Autodesk Inventor part; units mm, degrees
ref_plane "YZ Plane" through (0, 0, 0) normal (1, 0, 0) x (0, 1, 0)
ref_plane "XZ Plane" through (0, 0, 0) normal (0, 1, 0) x (-1, 0, 0)
ref_plane "XY Plane" through (0, 0, 0) normal (0, 0, 1) x (1, 0, 0)
sketch "Sketch1" plane through (0, 0, 0) normal (0, 0, 1) x (1, 0, 0)
  line L0 (13.4603, 15.4458) -> (13.4545, -36.9417)
  circle A0 centre (18.2181, -26.6234) radius 2.3812
  circle A1 centre (18.2217, 5.1266) radius 2.3812
  circle A2 centre (78.5467, 5.1199) radius 2.3812
  circle A3 centre (78.5431, -26.6301) radius 2.3812
  circle A4 centre (169.0306, -26.6401) radius 2.3812
  circle A5 centre (229.3556, -26.6468) radius 2.3812
  circle A6 centre (229.3592, 5.1032) radius 2.3812
  line L1 (234.1228, 15.4214) -> (234.117, -36.9661)
  circle A7 centre (169.0342, 5.1099) radius 2.3812
  line L2 (13.4545, -36.9417) -> (234.117, -36.9661)
  line L3 (234.1228, 15.4214) -> (13.4603, 15.4458)
  point P0 (3.3527, -2.3752)
extrude "Extrusion1" add sketch "Sketch1" along normal blind 12.7
sketch "Sketch3" plane through (0, 0, 0) normal (0, 0, -1) x (-1, 0, 0)
  line L0 (-234.117, -36.9661) -> (-234.1228, 15.4214)
  line L1 (-234.1199, -10.7723) -> (-13.4574, -10.7479)
  line L2 (-13.4603, 15.4458) -> (-13.4545, -36.9417)
  line L3 (-234.1228, 15.4214) -> (-13.4603, 15.4458)
  line L4 (-123.7915, 15.4336) -> (-123.7857, -36.9539)
  line L5 (-13.4545, -36.9417) -> (-234.117, -36.9661)
  circle A0 centre (-155.5369, -26.2636) radius 1.5
  circle A1 centre (-131.5369, -26.261) radius 1.5
  circle A2 centre (-155.5404, 4.7364) radius 1.5
  circle A3 centre (-131.5404, 4.739) radius 1.5
  point P0 (0, 0)
  dimension "d8" = 15.5
  dimension "d9" = 31.75
  dimension "d10" = 3
  dimension "d13" = 24
  dimension "d16" = 31
extrude "Extrusion2" cut sketch "Sketch3" against normal blind 12.7 contours A0 | A1 | A2 | A3
sketch "Sketch4" plane through (0, 0, 0) normal (0, 0, -1) x (-1, 0, 0)
  circle A0 centre (-131.5369, -26.261) radius 1.5
  circle A1 centre (-131.5369, -26.261) radius 3.175
  circle A2 centre (-155.5369, -26.2636) radius 1.5
  circle A3 centre (-155.5369, -26.2636) radius 3.175
  circle A4 centre (-131.5404, 4.739) radius 1.5
  circle A5 centre (-131.5404, 4.739) radius 3.175
  circle A6 centre (-155.5404, 4.7364) radius 1.5
  circle A7 centre (-155.5404, 4.7364) radius 3.175
  point P0 (0, 0)
  dimension "d21" = 6.35
  dimension "d22" = 6.35
  dimension "d23" = 6.35
  dimension "d24" = 6.35
extrude "Extrusion3" cut sketch "Sketch4" against normal blind 3.175
sketch "Sketch5" plane through (0, 0, 0) normal (0, 0, -1) x (-1, 0, 0)
  point P0 (0, 0)
sketch "Sketch6" plane through (0, 0, 0) normal (0, 0, -1) x (-1, 0, 0)
  point P0 (0, 0)
sketch "Sketch7" plane through (0, 0, 0) normal (0, 0, -1) x (-1, 0, 0)
  point P0 (0, 0)
sketch "Sketch8" plane through (0, 0, 0) normal (0, 0, -1) x (-1, 0, 0)
  circle A0 centre (-108.2333, 8.2916) radius 1.5875
  line L0 (-234.1228, 15.4214) -> (-13.4603, 15.4458) construction
  line L1 (-123.7915, 15.4336) -> (-123.7857, -36.9539) construction
  line L2 (-13.4545, -36.9417) -> (-234.117, -36.9661) construction
  line L3 (-234.117, -36.9661) -> (-234.1228, 15.4214) construction
  line L4 (-234.1199, -10.7723) -> (-13.4574, -10.7479) construction
  line L5 (-13.4603, 15.4458) -> (-13.4545, -36.9417) construction
  circle A1 centre (-108.229, -29.8084) radius 1.5875
  circle A2 centre (-139.9833, 8.2881) radius 1.5875
  circle A3 centre (-139.979, -29.8119) radius 1.5875
  point P0 (0, 0)
  dimension "d27" = 3.175
  dimension "d28" = 15.5575
  dimension "d31" = 38.1
  dimension "d34" = 31.75
  dimension "d37" = 19.05
extrude "Extrusion4" cut sketch "Sketch8" against normal blind 25.4
sketch "Sketch9" plane through (0, 0, 12.7) normal (0, 0, 1) x (1, 0, 0)
  circle A0 centre (155.5369, -26.2636) radius 1.5
  circle A1 centre (131.5369, -26.261) radius 1.5
  circle A2 centre (155.5404, 4.7364) radius 1.5
  circle A3 centre (131.5404, 4.739) radius 1.5
  circle A4 centre (155.5369, -26.2636) radius 3.175
  circle A5 centre (131.5369, -26.261) radius 3.175
  circle A6 centre (131.5404, 4.739) radius 3.175
  circle A7 centre (155.5404, 4.7364) radius 3.175
  point P0 (0, 0)
  dimension "d40" = 6.35
  dimension "d41" = 6.35
  dimension "d42" = 6.35
  dimension "d43" = 6.35
extrude "Extrusion5" cut sketch "Sketch9" against normal blind 3.175
sketch "Sketch10" plane through (0, 0, 0) normal (0, 0, -1) x (-1, 0, 0)
  circle A0 centre (-88.9984, 1.2723) radius 3.175
  circle A1 centre (-88.9953, -22.4777) radius 3.175
  circle A2 centre (-88.9953, -22.4777) radius 3.9688
  circle A3 centre (-88.9984, 1.2723) radius 3.9688
  point P0 (0, 0)
  dimension "d46" = 7.9375
  dimension "d47" = 7.9375
extrude "Extrusion6" cut sketch "Sketch10" against normal blind 12.7 contours A0 | A1 | A2 | A3
fillet "Fillet1" radius 0.254 4 edges at (92.9672, 1.2723, 12.7) (92.9641, -22.4777, 12.7) (92.9641, -22.4777, 0) (92.9672, 1.2723, 0)
sketch "Sketch11" plane through (0, 0, 0) normal (0, 0, -1) x (-1, 0, 0)
  circle A0 centre (-88.9953, -22.4777) radius 3.9688
  circle A1 centre (-139.979, -29.8119) radius 1.5875
  circle A2 centre (-139.9833, 8.2881) radius 1.5875
  circle A3 centre (-108.229, -29.8084) radius 1.5875
  circle A4 centre (-108.2333, 8.2916) radius 1.5875
  circle A5 centre (-155.5404, 4.7364) radius 3.175
  circle A6 centre (-155.5369, -26.2636) radius 3.175
  circle A7 centre (-131.5404, 4.739) radius 3.175
  circle A8 centre (-131.5369, -26.261) radius 3.175
  line L0 (-13.4545, -36.9417) -> (-234.117, -36.9661)
  line L1 (-13.4603, 15.4458) -> (-13.4545, -36.9417)
  line L2 (-234.1228, 15.4214) -> (-13.4603, 15.4458)
  line L3 (-234.117, -36.9661) -> (-234.1228, 15.4214)
  circle A9 centre (-169.0342, 5.1099) radius 2.3812
  circle A10 centre (-229.3592, 5.1032) radius 2.3812
  circle A11 centre (-229.3556, -26.6468) radius 2.3812
  circle A12 centre (-169.0306, -26.6401) radius 2.3812
  circle A13 centre (-78.5431, -26.6301) radius 2.3812
  circle A14 centre (-78.5467, 5.1199) radius 2.3812
  circle A15 centre (-18.2217, 5.1266) radius 2.3812
  circle A16 centre (-18.2181, -26.6234) radius 2.3812
  circle A17 centre (-88.9984, 1.2723) radius 4.2227
  point P0 (0, 0)
  dimension "d51" = 10.3187
  dimension "d53" = 4.7625
  dimension "d54" = 220.6625
  dimension "d55" = 4.7625
  dimension "d56" = 65.0875
  dimension "d57" = 94.7738
  dimension "d58" = 118.0812
  dimension "d59" = 7.9375
  dimension "d60" = 126.5238
  dimension "d61" = 142.0813
  dimension "d62" = 155.575
  dimension "d63" = 215.9
  dimension "d64" = 14.4724
  dimension "d65" = 42.0688
  dimension "d66" = 7.1437
  dimension "d67" = 38.2224
  dimension "d68" = 10.6937
  dimension "d69" = 45.2437
  dimension "d70" = 41.6938
  dimension "d71" = 52.3875
properties part number "Head Adapter Plate"
Build history of the part. All positions in model axes, mm. A direction names the side the tool comes from. Round coordinates to 2 decimals unless told otherwise and drop trailing zeros. One line per item, written item: value. Start each with the question number.
Q1. Drop flat-ended pins along their axis: pin 1 Ø1.9 at (x, y) = (132.5, -27) entering from -Z (3 decimals); pin 2 Ø10 at (x, y) = (155.54, -26.26) entering from -Z; pin 3 Ø4 at (y, z) = (-19.5, 5.5) entering from +X; pin 4 Ø1.9 at (x, y) = (157, 4) entering from +Z (3 decimals). Give the stop position or say it passes through.
Q2. Probe line 1 along Y through (x, z) = (156.5, 6.75); line 2 along Y through (x, z) = (90.5, 3.25); line 3 along X through (y, z) = (-28, 6.25). List the from-to ranges inside material, lowest first.
Q3. 3-axis set-ups, long thin cutter, end or side, ignore diameter. For faces 3 (the face through (80.818, 4.405, 6.261)), 4 (the face through (134.06, 2.81, 1.57)), 5 (the face through (132, -28, 9.525)): which of +Z, -Z, +X, -X, +Y, -Y reach the whole face in a straight line?
Q4. Two-plate mould, pull along X, no slides. Class faces 1 (the face through (122, -10, 12.7)), 2 (the face through (171.305, 4.395, 6.261)): released by +X, released by -X, zero draft, split by the parting line, or undercut.
Q5. Cut at A-A on z = 5.5. Count the separate pieces of the cut face and the enclosed holes in it, plus the area to 3 significant figures.
Computed:
1. pin 1: z = 3.175
1. pin 2: z = 0
1. pin 3: x = 234.12
1. pin 4: z = 9.525
2. line 1: -36.96 to -27.41, -25.11 to 3.58, 5.89 to 15.43
2. line 2: -36.95 to -26.15, -18.81 to -2.4, 4.95 to 15.44
2. line 3: 13.46 to 16.28, 20.16 to 76.6, 80.49 to 167.08, 170.99 to 227.4, 231.31 to 234.12
3. face 3: +Z, -Z
3. face 4: -Z
3. face 5: +Z
4. face 1: zero draft
4. face 2: undercut
5. separate pieces: 1
5. enclosed holes: 18
5. area: 11,300 mm²
